Autodesk Inventor part; units mm, degrees
ref_plane "YZ Plane" through (0, 0, 0) normal (1, 0, 0) x (0, 1, 0)
ref_plane "XZ Plane" through (0, 0, 0) normal (0, 1, 0) x (-1, 0, 0)
ref_plane "XY Plane" through (0, 0, 0) normal (0, 0, 1) x (1, 0, 0)
sketch "Sketch1" plane through (0, 0, 0) normal (1, 0, 0) x (0, 1, 0)
  line L0 (0, 0) -> (0, -90)
  line L1 (0, -90) -> (7.5, -90)
  line L2 (7.5, -90) -> (7.5, -60)
  line L3 (7.5, -60) -> (20, -60)
  line L4 (20, -60) -> (20, -40)
  line L5 (20, -40) -> (30, -40)
  line L6 (30, -40) -> (30, -20)
  line L7 (30, -20) -> (45, -20)
  line L8 (45, -20) -> (45, 0)
  line L9 (45, 0) -> (0, 0)
  dimension "d0" = 90
  dimension "d1" = 15
  dimension "d2" = 40
  dimension "d3" = 60
  dimension "d4" = 90
  dimension "d5" = 20
  dimension "d6" = 20
  dimension "d7" = 20
revolve "Revolution1" add sketch "Sketch1" angle 360 about axis through (0, 0, 0) along (0, 0, -1)
Design review of the part built by this model. Coordinates are the model's own, in mm. A direction names the side the tool comes from. Coordinates: 2 decimals unless noted, no trailing zeros. Loops run counter-clockwise (first coordinate to the right, second up) from the corner with the lowest first, then second, coordinate; pieces in that order, holes last. Notation, with made-up numbers: (-3, 52.5) - (9, 52.5) arc R20 cw to (9, 82.5) - close; hole circle Ø4 at (-16.5, 1). An arc over 180 degrees is marked (long way). Use CSV: the item, a comma, the result in double quotes. Start each with the question number.
1. Add section D-D on y = -27.5. Give the boundary of the cut face in (x, z).
2. Add section C-C on z = -43.5. Give the boundary of the cut face in (x, y).
3. Clearance check with flat-ended pins moving along their axes: pin 1 (3 mm diameter, centred on x = -4, z = -20.5, fed in from +Y); pin 2 (2 mm diameter, centred on x = -21.5, y = 30.5, fed in from -Z); pin 3 (5 mm diameter, centred on x = 17.5, y = -22.5, fed in from -Z). State where each tip first meets the part, or that it passes through.
4. Add section A-A on x = 0. Give the boundary of the cut face in (y, z).
5. To check wall thickness, follow probe 1 along Z at (x, y) = (-25, -23.5); probe 2 along Z at (x, y) = (-27, -5.5); probe 3 along X at (y, z) = (-1, -42.5). State the ranges of each line that lie inside material, in increasing order.
6. For faces 1 (the cylindrical face through (-0.33, -7.493, -74.79)), 2 (the cylindrical face through (39.923, 20.765, -9.86)), list the 3-axis set-ups (+Z, -Z, +X, -X, +Y, -Y) from which the entire face can be reached by the end or side of a thin tool; tool diameter is ignored.
Resolved:
1,outline,"(-35.62, -20) - (-11.99, -20) - (-11.99, -40) - (11.99, -40) - (11.99, -20) - (35.62, -20) - (35.62, 0) - (-35.62, 0) - close"
2,outline,"circle Ø40 at (0, 0)"
3,pin 1,"y = 44.93"
3,pin 2,"z = -20"
3,pin 3,"z = -40"
4,outline,"(-45, -20) - (-30, -20) - (-30, -40) - (-20, -40) - (-20, -60) - (-7.5, -60) - (-7.5, -90) - (7.5, -90) - (7.5, -60) - (20, -60) - (20, -40) - (30, -40) - (30, -20) - (45, -20) - (45, 0) - (-45, 0) - close"
5,probe 1,"-20 to 0"
5,probe 2,"-40 to 0"
5,probe 3,"-19.97 to 19.97"
6,face 1,"-Z"
6,face 2,"+Z, -Z"
